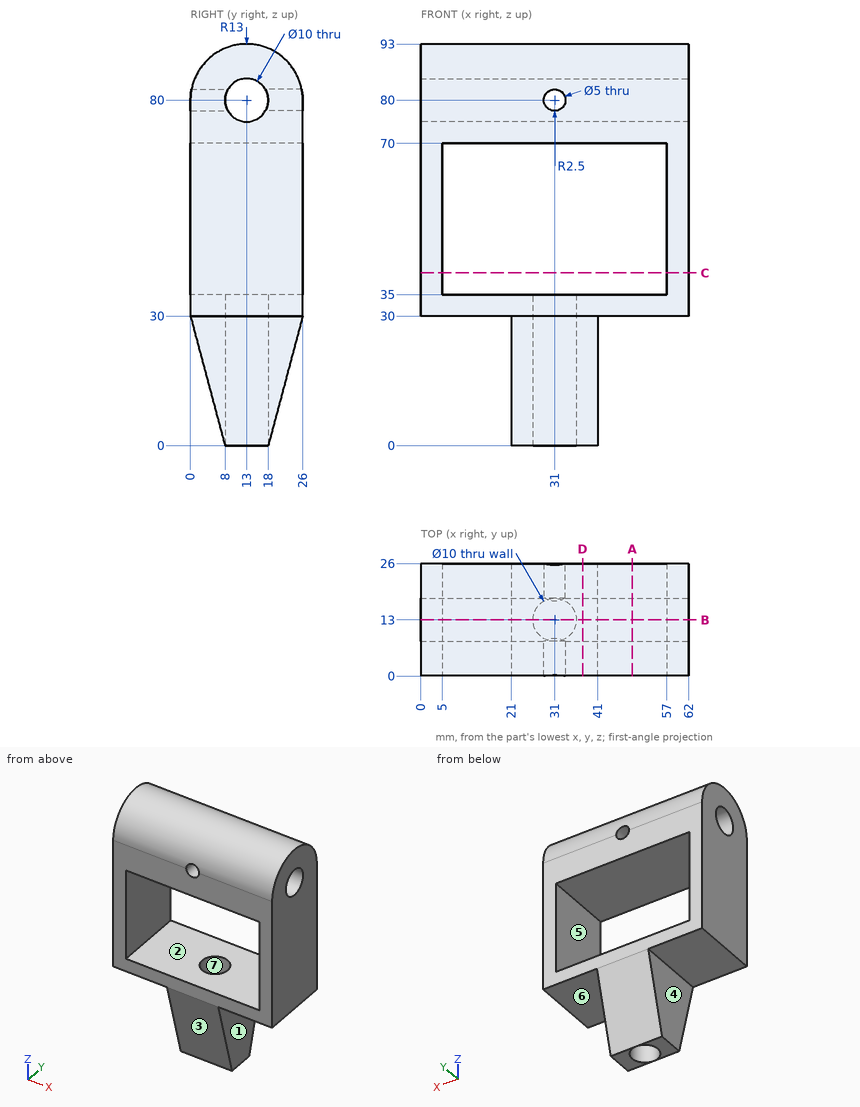
Input: dimensioned drawing with shaded views. Units: mm. Origin: part minimum x, y, z. A direction names the side the tool comes from. Round coordinates to 2 decimals unless told otherwise and drop trailing zeros. Loops run counter-clockwise (first coordinate to the right, second up) from the corner with the lowest first, then second, coordinate; pieces in that order, holes last. Notation, with made-up numbers: (-19.75, -17.75) -> (7.25, -17.75) arc R24 cw to (7.25, 18.25) -> close; hole circle Ø2 at (3, 61.5). An arc over 180 degrees is marked (long way). Use one line per item in the form item = value. Start each with the question number.
1) Access query for the marked faces 4, 5, 6 and 7. Directions: +Z, -Z, +X, -X, +Y, -Y. A direction counts if a zero-diameter tool reaches every point of the face in a straight line with its end or side. Return the directions, or none.
2) First-contact query: P1, Ø10, axis at x = 39.5, y = 20, coming from the +Z side; P2, Ø6, axis at y = 13, z = 80, coming from the -X side; P3, Ø1, axis at x = 24.5, y = 10.5, coming from the -Z side; P4, Ø3, axis at y = 5, z = 26, coming from the -X side. Flat tips, straight axial feed; report the tip coordinate or a pass-through.
3) Section D-D on x = 37.5. Output: boundary loops of the cut face in (y, z), then the cut area to 3 significant figures.
4) Draft query along X for the marked faces 1, 2 and 3. Return one class per face: released by +X, released by -X, zero draft, split by the parting line, or undercut.
5) Section A-A on x = 49. Output: boundary loops of the cut face in (y, z).
6) Line query: L1, parallel to X at y = 18.75, z = 40.5; L2, parallel to Z at x = 19.5, y = 15.5; L3, parallel to Z at x = 46.5, y = 17.5. Output: solid intervals per line, ascending.
7) Section C-C on z = 40. Output: boundary loops of the cut face in (x, y).
8) Section B-B on y = 13. Output: boundary loops of the cut face in (x, z), then the cut area to 3 significant figures.
Response:
q1.face_4 = -Z, -X, +Y, -Y
q1.face_5 = +Y, -Y
q1.face_6 = -Z, +X, +Y, -Y
q1.face_7 = -Z
q2.P1 = 92.85
q2.P2 = through
q2.P3 = 0
q2.P4 = 21
q3.outline = (0, 30) -> (8, 0) -> (18, 0) -> (26, 30) -> (26, 35) -> (0, 35) -> close; (0, 70) -> (26, 70) -> (26, 80) arc R13 ccw to (0, 80) -> close; hole circle Ø10 at (13, 80)
q3.area = 1,120 mm^2
q4.face_1 = released by +X
q4.face_2 = undercut
q4.face_3 = zero draft
q5.outline = (0, 30) -> (26, 30) -> (26, 35) -> (0, 35) -> close; (0, 70) -> (26, 70) -> (26, 80) arc R13 ccw to (0, 80) -> close; hole circle Ø10 at (13, 80)
q6.L1 = 0 to 5, 57 to 62
q6.L2 = 30 to 35, 70 to 75.67, 84.33 to 92.76
q6.L3 = 30 to 35, 70 to 77.82, 82.18 to 92.2
q7.outline = (0, 0) -> (5, 0) -> (5, 26) -> (0, 26) -> close; (57, 0) -> (62, 0) -> (62, 26) -> (57, 26) -> close
q8.outline = (0, 30) -> (21, 30) -> (21, 0) -> (26, 0) -> (26, 35) -> (5, 35) -> (5, 70) -> (57, 70) -> (57, 35) -> (36, 35) -> (36, 0) -> (41, 0) -> (41, 30) -> (62, 30) -> (62, 75) -> (0, 75) -> close; (0, 85) -> (62, 85) -> (62, 93) -> (0, 93) -> close
q8.area = 1,720 mm^2
